Here's how the part is built. I have some questions about the finished solid (model axes, mm). A direction names the side the tool comes from. Coordinates: 2 decimals unless noted, no trailing zeros. Loops run counter-clockwise (first coordinate to the right, second up) from the corner with the lowest first, then second, coordinate; pieces in that order, holes last. Notation, with made-up numbers: (70.25, 55) -> (96.25, 55) arc R30 cw to (96.25, 78) -> close; hole circle Ø9 at (-4, 28). An arc over 180 degrees is marked (long way). Answer as a JSON object with one key per item and string values. Group by question number.
1) If we mould it in two halves opening along Y, with no side actions, what happens to faces 4 (the cylindrical face through (9.45, -69.36, 3.94)), 5 (the flat face through (8.55, -78, 4)), 6 (the cylindrical face through (0.193, -68.604, 4.056))? For each: +Y half, -Y half, draft (parallel to the pull), parting line (faces both ways), or undercut.
2) I want a section at D-D (y = 30). Write out the boundary of the cut face in (x, z), then the cut area to 3 significant figures.
3) I want a section at A-A (z = 4). Count the separate pieces of the cut face and the enclosed holes in it, then the cut area to 3 significant figures.
4) I need wall thicknesses on probe 1 along X at (y, z) = (-73.5, 4.25); probe 2 along Y at (x, z) = (-4, 5.75); probe 3 along Y at (x, z) = (-2, 1.5). Which ranges of each line are inside material? Lowest first, please. Write a range as [from, to].
5) Which directions (+Z, -Z, +X, -X, +Y, -Y) give clear straight access to the entire face, cutting with the end or side of a thin tool? Please do faces 1 (the flat face through (-1.55, -83, 4)), 2 (the flat face through (13, -68.5, 4)), 3 (the flat face through (-5, -86.5, 4)).
6) I want a section at B-B (y = -80.5). Write out the boundary of the cut face in (x, z).
7) I'm going to push flat-ended pins straight in: pin 1 (3 mm diameter, centred on y = -66, z = 3.5, fed in from -X); pin 2 (2 mm diameter, centred on y = 8, z = 4, fed in from -X); pin 3 (2.5 mm diameter, centred on y = -82, z = 4.5, fed in from -X). Where does each tip first touch, or does it pass through?
8) I want a section at C-C (y = -11). Write out the boundary of the cut face in (x, z), then the cut area to 3 significant figures.
```python
from build123d import *

# Parameters (mm, degrees)
SKETCH1_W           = 32
SKETCH1_H           = 173
BOSS_EXTRUDE2_DEPTH = 8
SKETCH3_R           = 4.9
SKETCH3_R_2         = 3
SKETCH3_W           = 3.1
SKETCH3_H           = 8.35
CUT_EXTRUDE1_DEPTH  = 9
CUT_EXTRUDE4_DEPTH  = 9
FILLET1_R           = 1
FILLET3_R           = 1
FILLET5_R           = 3
FILLET6_R           = 0.5
SKETCH7_R           = 2
CUT_EXTRUDE5_DEPTH  = 25.1


with BuildPart() as part:
    # Sketch1 → Boss-Extrude2 (new body)
    with BuildSketch(Plane.XY):
        Rectangle(SKETCH1_W, SKETCH1_H)
    extrude(amount=BOSS_EXTRUDE2_DEPTH)

    # Sketch3 → Cut-Extrude1 (cut, through all)
    with BuildSketch(Plane.XY.offset(8)):
        with Locations((0, -73.5)):
            Circle(SKETCH3_R)
        with Locations((0, 76.5)):
            Circle(SKETCH3_R_2)
        with Locations((0, -82.325)):
            Rectangle(SKETCH3_W, SKETCH3_H)
    extrude(amount=-CUT_EXTRUDE1_DEPTH, mode=Mode.SUBTRACT)

    # Sketch5 → Cut-Extrude4 (cut, through all)
    with BuildSketch(Plane.XY.offset(8)):
        with BuildLine():
            Line((-16, 86.5), (-16, -86.5))
            Line((-16, -86.5), (-15.540973095, -74.029769072))
            ThreePointArc((-15.540973095, -74.029769072), (-15.53947586, -72.927994754), (-15.459966578, -71.829092044))
            Line((-15.459966578, -71.829092044), (-10, 76.5))
            ThreePointArc((-10, 76.5), (-7.07106782, 83.571067803), (-2.4e-08, 86.5))
            Line((-2.4e-08, 86.5), (-16, 86.5))
        make_face()
        with BuildLine():
            Line((16, 86.5), (-2.4e-08, 86.5))
            ThreePointArc((-2.4e-08, 86.5), (6.939944042, 83.699803935), (9.993247284, 76.867435316))
            Line((9.993247284, 76.867435316), (15.338169515, -68.5))
            Line((15.338169515, -68.5), (8.55, -68.5))
            Line((8.55, -68.5), (8.55, -86.5))
            Line((8.55, -86.5), (16, -86.5))
            Line((16, -86.5), (16, 86.5))
        make_face()
        with BuildLine():
            Line((-15.540973095, -74.029769072), (-16, -86.5))
            Line((-16, -86.5), (-8.532438104, -86.5))
            ThreePointArc((-8.532438104, -86.5), (-13.555771706, -81.118631994), (-15.540973095, -74.029769072))
        make_face()
    extrude(amount=-CUT_EXTRUDE4_DEPTH, mode=Mode.SUBTRACT)

    # Fillet1
    fillet1_edges = [part.edges().sort_by_distance(p)[0] for p in [
        (8.55, -86.5, 4),
    ]]
    fillet(fillet1_edges, radius=FILLET1_R)

    # Fillet3
    fillet3_edges = [part.edges().sort_by_distance(p)[0] for p in [
        (15.338169515, -68.5, 4),
    ]]
    fillet(fillet3_edges, radius=FILLET3_R)

    # Fillet5
    fillet5_edges = [part.edges().sort_by_distance(p)[0] for p in [
        (8.55, -68.5, 4),
    ]]
    fillet(fillet5_edges, radius=FILLET5_R)

    # Fillet6
    fillet6_edges = [part.edges().sort_by_distance(p)[0] for p in [
        (-8.532438104, -86.5, 4),
    ]]
    fillet(fillet6_edges, radius=FILLET6_R)

    # Sketch7 → Cut-Extrude5 (cut, through all)
    with BuildSketch(Plane(origin=(8.55, 0, 0), x_dir=(0, 0, -1), z_dir=(1, 0, 0))):
        with Locations((-4, -80.5)):
            Circle(SKETCH7_R)
    extrude(amount=-CUT_EXTRUDE5_DEPTH, mode=Mode.SUBTRACT)


solid = part.part
```
Determined:
{
 "1": {"face 4": "-Y half", "face 5": "draft", "face 6": "undercut"},
 "2": {"outline": "(-11.71, 0) -> (11.72, 0) -> (11.72, 8) -> (-11.71, 8) -> close", "area": "187 mm^2"},
 "3": {"separate pieces": "3", "enclosed holes": "1", "area": "4,030 mm^2"},
 "4": {"probe 1": "[-15.55, -4.9], [4.9, 8.55]", "probe 2": "[-86.5, -81.47], [-79.53, -76.33], [-70.67, 85.67]", "probe 3": "[-86.5, -77.97], [-69.03, 74.26], [78.74, 86.3]"},
 "5": {"face 1": "+Z, -Z, -Y", "face 2": "+Z, -Z, +X, -Y", "face 3": "+Z, -Z, +X, -X, -Y"},
 "6": {"outline": "(-13.89, 0) -> (-1.55, 0) -> (-1.55, 2) -> (-13.89, 2) -> close; (-13.89, 6) -> (-1.55, 6) -> (-1.55, 8) -> (-13.89, 8) -> close; (1.55, 0) -> (8.55, 0) -> (8.55, 2) -> (1.55, 2) -> close; (1.55, 6) -> (8.55, 6) -> (8.55, 8) -> (1.55, 8) -> close"},
 "7": {"pin 1": "x = -15.3", "pin 2": "x = -12.56", "pin 3": "x = -13.28"},
 "8": {"outline": "(-13.22, 0) -> (13.22, 0) -> (13.22, 8) -> (-13.22, 8) -> close", "area": "212 mm^2"}
}
